Build history of the part. All positions in model axes, mm. A direction names the side the tool comes from. Give positions to 0.01 mm unless a question says otherwise; leave off trailing zeros. Order: outer loops, then holes, each group sorted by start corner. A loop starts at its lowest first (then second) coordinate and runs counter-clockwise, first axis right, second up. Notation, with made-up numbers: (86.5, -27.75) - (138.5, -27.75) arc R9 cw to (138.5, -15.75) - close; hole circle Ø1 at (-28, 28). An arc over 180 degrees is marked (long way). Use a Markdown table: item, result.
from build123d import *

# Parameters (mm, degrees)
PAD003_DEPTH    = 12.5
POCKET006_DEPTH = 182.8372896975
POCKET007_DEPTH = 24.5
CHAMFER002_SIZE = 3


with BuildPart() as part:
    # Sketch011 → Pad003 (new body, symmetric)
    with BuildSketch(Plane.XY):
        with BuildLine():
            ThreePointArc((0, 19.5), (-13.7885822331, 13.7885822331), (-19.5, 0))
            Line((-32.5, 0), (-19.5, 0))
            ThreePointArc((-8, 31.5), (-25.6539470647, 19.9530699392), (-32.5, 0))
            Line((0, 31.5), (-8, 31.5))
            Line((0, 31.5), (0, 19.5))
        make_face()
    pad003 = extrude(amount=PAD003_DEPTH, both=True)

    # Mirrored004: Pad003 across Sketch011 H_Axis
    add(pad003.mirror(Plane.ZX))

    # Sketch012 (on Face1 of Mirrored004) → Pocket006 (cut, through all)
    with BuildSketch(Plane.YZ):
        with BuildLine():
            ThreePointArc((26.75, -2.918582704), (25.5, 3.175), (24.25, -2.918582704))
            Line((24.25, -2.918582704), (24.65, -3.318582704))
            Line((24.65, -3.318582704), (26.35, -3.318582704))
            Line((26.35, -3.318582704), (26.75, -2.918582704))
        make_face()
    pocket006 = extrude(amount=-POCKET006_DEPTH, mode=Mode.SUBTRACT)

    # Mirrored005: Pocket006 across Sketch012 V_Axis
    add(pocket006.mirror(Plane(origin=(0, 0, 0), x_dir=(1, 0, 0), z_dir=(0, 1, 0))), mode=Mode.SUBTRACT)

    # Sketch013 (on DatumPlane) → Pocket007 (cut)
    with BuildSketch(Plane(origin=(-34, 0, 0), x_dir=(0, -1, 0), z_dir=(-1, 0, 0))):
        Polygon((-19.9, 3.2331615075), (-25.5, 6.4663230149), (-31.1, 3.2331615075), (-31.1, -3.2331615075), (-25.5, -6.4663230149), (-19.9, -3.2331615075), align=None)
    pocket007 = extrude(amount=-POCKET007_DEPTH, mode=Mode.SUBTRACT)

    # Mirrored006: Pocket007 across Sketch013 V_Axis
    add(pocket007.mirror(Plane(origin=(-34, 0, 0), x_dir=(-1, 0, 0), z_dir=(0, -1, 0))), mode=Mode.SUBTRACT)

    # Chamfer002
    chamfer002_edges = [part.edges().sort_by_distance(p)[0] for p in [
        (-4, -31.5, -12.5),
        (-25.653947, -19.95307, -12.5),
        (-25.653947, 19.95307, -12.5),
        (-4, 31.5, -12.5),
    ]]
    chamfer(chamfer002_edges, length=CHAMFER002_SIZE)


solid = part.part
1) Slice it at A-A (z = 0). Write the cut outline in (x, y) (3 decimals), and give its area (3 significant figures).
Computed:
| item | result |
|---|---|
| outline | (-25.695, -19.9) - (-9.5, -19.9) - (-9.5, -22.325) - (0, -22.325) - (0, -19.5) arc R19.5 cw to (0, 19.5) - (0, 22.325) - (-9.5, 22.325) - (-9.5, 19.9) - (-25.695, 19.9) arc R32.5 ccw to start; (-9.5, -31.081) arc R32.5 ccw to (-8, -31.5) - (0, -31.5) - (0, -28.675) - (-9.5, -28.675) - close; (-9.5, 28.675) - (0, 28.675) - (0, 31.5) - (-8, 31.5) arc R32.5 ccw to (-9.5, 31.081) - close |
| area | 709 mm² |
2) Slice it at B-B (z = -8.5). Write the cut outline in (x, y), and give its area (3 significant figures).
Computed:
| item | result |
|---|---|
| outline | (-8, -31.5) - (0, -31.5) - (0, -19.5) arc R19.5 cw to (0, 19.5) - (0, 31.5) - (-8, 31.5) arc R32.5 ccw to start |
| area | 1,050 mm² |
3) Wall check: line 1 (Y direction, x = -6, z = 0) (3 decimals); line 2 (Z direction, x = -4.75, y = 25.5) (3 decimals); line 3 (Y direction, x = -4, z = 0.5). Give the ranges that are in metal, low to high. Write a range as from..to.
Computed:
| item | result |
|---|---|
| line 1 | y = -31.5..-28.675, -22.325..-18.554, 18.554..22.325, 28.675..31.5 |
| line 2 | z = -12.5..-3.319, 3.175..12.5 |
| line 3 | y = -31.5..-28.64, -22.36..-19.09, 19.09..22.36, 28.64..31.5 |
4) Slice it at C-C (z = -5.5). Write the cut outline in (x, y), and give its area (3 significant figures).
Computed:
| item | result |
|---|---|
| outline | (-22.1, -23.83) - (-9.5, -23.83) - (-9.5, -27.17) - (-17.83, -27.17) arc R32.5 ccw to (-8, -31.5) - (0, -31.5) - (0, -19.5) arc R19.5 cw to (0, 19.5) - (0, 31.5) - (-8, 31.5) arc R32.5 ccw to (-17.83, 27.17) - (-9.5, 27.17) - (-9.5, 23.83) - (-22.1, 23.83) arc R32.5 ccw to start |
| area | 980 mm² |
5) Two-plate mould, pull along Z, no slides. Class faces 4 (the flat face through (0, -24, 3)), 5 (the flat face through (-15.911, 22.661, 4.827)), 6 (the flat face through (-20, 0, 12.5)), 7 (the flat face through (-21, 0, -12.5)): +Z half, -Z half, draft (parallel to the pull), parting line (faces both ways), or undercut.
Computed:
| item | result |
|---|---|
| face 4 | draft |
| face 5 | undercut |
| face 6 | +Z half |
| face 7 | -Z half |
6) Pin check, flat tips, straight feed: P1, Ø5.5, axis at y = -24.5, z = 1.5, coming from the -X side; P2, Ø1, axis at x = -27, z = 1, coming from the +Y side; P3, Ø6, axis at y = 2.5, z = -2.5, coming from the +X side; P4, Ø5, axis at y = -25.5, z = 0, coming from the +X side. Stop position of each tip, or through.
Computed:
| item | result |
|---|---|
| P1 | stops at x = -9.5 |
| P2 | stops at y = 18.81 |
| P3 | stops at x = -18.71 |
| P4 | passes through |
7) Tool access for faces 1 (the flat face through (-5, -25, -3.319)), 2 (the flat face through (-18, 19.9, 0)), 3 (the flat face through (-9.5, 27, 3)): list every direction of +Z, -Z, +X, -X, +Y, -Y with a clear straight run to the whole face (end or side of a thin tool).
Computed:
| item | result |
|---|---|
| face 1 | +X, -X |
| face 2 | -X, +Y |
| face 3 | -X |
